from build123d import *

# Parameters (mm, degrees)
SKETCH_W        = 90
SKETCH_H        = 40
PAD_DEPTH       = 11
POCKET_DEPTH    = 9
POCKET001_DEPTH = 6
SKETCH003_W     = 13.5
SKETCH003_H     = 3.4
POCKET002_DEPTH = 6
SKETCH005_R     = 3
HOLE_DEPTH      = 25
FILLET_R        = 1
FILLET001_R     = 2.5
SKETCH007_W     = 6
SKETCH007_H     = 6
POCKET003_DEPTH = 1
FILLET002_R     = 1


with BuildPart() as part:
    # Sketch → Pad (new body)
    with BuildSketch(Plane.XY):
        with Locations((45, 20)):
            Rectangle(SKETCH_W, SKETCH_H)
    extrude(amount=PAD_DEPTH)

    # Sketch001 (on Face6 of Pad) → Pocket (cut)
    with BuildSketch(Plane.XY.offset(11)):
        Polygon((4.5, 30.5), (4.5, 9.5), (9.5, 9.5), (9.5, 4.5), (80.5, 4.5), (80.5, 9.5), (85.5, 9.5), (85.5, 30.5), (80.5, 30.5), (80.5, 35.5), (9.5, 35.5), (9.5, 30.5), align=None)
    extrude(amount=-POCKET_DEPTH, mode=Mode.SUBTRACT)

    # Sketch002 (on Face6 of Pocket) → Pocket001 (cut)
    with BuildSketch(Plane.YZ.offset(90)):
        with BuildLine():
            ThreePointArc((17.5, 11), (20, 8.499988), (22.5, 11))
            Line((17.5, 11), (22.5, 11))
        make_face()
    extrude(amount=-POCKET001_DEPTH, mode=Mode.SUBTRACT)

    # Sketch003 (on Face1 of Pocket001) → Pocket002 (cut)
    with BuildSketch(Plane(origin=(0, 0, 0), x_dir=(0, -1, 0), z_dir=(-1, 0, 0))):
        with Locations((-18.75, 9.3)):
            Rectangle(SKETCH003_W, SKETCH003_H)
    extrude(amount=-POCKET002_DEPTH, mode=Mode.SUBTRACT)

    # Sketch005 (on Face8 of Pocket002) → Hole (cut)
    with BuildSketch(Plane.XY.offset(11)):
        with Locations((4.5, 35.5)):
            Circle(SKETCH005_R)
        with Locations((4.5, 4.5)):
            Circle(SKETCH005_R)
        with Locations((85.5, 35.5)):
            Circle(SKETCH005_R)
        with Locations((85.5, 4.5)):
            Circle(SKETCH005_R)
    extrude(amount=-HOLE_DEPTH, mode=Mode.SUBTRACT)

    # Fillet
    fillet_edges = [part.edges().sort_by_distance(p)[0] for p in [
        (9.5, 30.5, 6.5),
        (80.5, 30.5, 6.5),
        (9.5, 9.5, 6.5),
        (80.5, 9.5, 6.5),
    ]]
    fillet(fillet_edges, radius=FILLET_R)

    # Fillet001
    fillet001_edges = [part.edges().sort_by_distance(p)[0] for p in [
        (0, 40, 5.5),
        (90, 40, 5.5),
        (90, 0, 5.5),
        (0, 0, 5.5),
    ]]
    fillet(fillet001_edges, radius=FILLET001_R)

    # Sketch007 (on Face25 of Fillet001) → Pocket003 (cut)
    with BuildSketch(Plane.XY.offset(2)):
        with Locations((45, 20)):
            Rectangle(SKETCH007_W, SKETCH007_H)
    extrude(amount=-POCKET003_DEPTH, mode=Mode.SUBTRACT)

    # Fillet002
    fillet002_edges = [part.edges().sort_by_distance(p)[0] for p in [
        (48, 23, 1.5),
        (42, 23, 1.5),
        (42, 17, 1.5),
        (48, 17, 1.5),
    ]]
    fillet(fillet002_edges, radius=FILLET002_R)


solid = part.part
The model under review builds one solid part; all positions refer to its coordinate system, in mm. A direction names the side the tool comes from. Round coordinates to 2 decimals unless told otherwise and drop trailing zeros. Write each loop counter-clockwise with the first axis right and the second up, starting at its lowest first coordinate (ties: lowest second). Pieces come first, ordered by that corner, then holes. Notation, with made-up numbers: (87.5, 64) -> (95.5, 64) arc R17 cw to (95.5, 78) -> close; hole circle Ø5 at (78, -16.75). An arc over 180 degrees is marked (long way). Answer as a JSON object with one key per item and string values.
1. We need section D-D on z = 10. State how many separate pieces and enclosed holes the cut face has, and give its area (3 significant figures).
Results found:
{"separate pieces": "2", "enclosed holes": "4", "area": "988 mm^2"}
2. We need section A-A on z = 4.75. State the section outline as (x, y) points, and give its area (3 significant figures).
Results found:
{"outline": "(0, 2.5) arc R2.5 ccw to (2.5, 0) -> (87.5, 0) arc R2.5 ccw to (90, 2.5) -> (90, 37.5) arc R2.5 ccw to (87.5, 40) -> (2.5, 40) arc R2.5 ccw to (0, 37.5) -> close; hole circle Ø6 at (4.5, 4.5); hole circle Ø6 at (4.5, 35.5); hole (4.5, 9.5) -> (8.5, 9.5) arc R1 cw to (9.5, 8.5) -> (9.5, 4.5) -> (80.5, 4.5) -> (80.5, 8.5) arc R1 cw to (81.5, 9.5) -> (85.5, 9.5) -> (85.5, 30.5) -> (81.5, 30.5) arc R1 cw to (80.5, 31.5) -> (80.5, 35.5) -> (9.5, 35.5) -> (9.5, 31.5) arc R1 cw to (8.5, 30.5) -> (4.5, 30.5) -> close; hole circle Ø6 at (85.5, 4.5); hole circle Ø6 at (85.5, 35.5)", "area": "1,070 mm^2"}
3. Machinability: for faces 4 (the face through (2, 25.5, 9)), 5 (the face through (89.248, 39.287, 5.577)), 6 (the face through (83, 9.5, 7)), which of the approach directions +Z, -Z, +X, -X, +Y, -Y give a long, thin tool a straight path to every point of the face, cutting with its end or side? Answer none if there is none.
Results found:
{"face 4": "+Z, -X", "face 5": "+Z, -Z, +X, +Y", "face 6": "+Z"}
4. We need section B-B on y = 20. State the section outline as (x, z) points.
Results found:
{"outline": "(0, 0) -> (90, 0) -> (90, 8.5) -> (85.5, 8.5) -> (85.5, 2) -> (48, 2) -> (48, 1) -> (42, 1) -> (42, 2) -> (4.5, 2) -> (4.5, 7.6) -> (0, 7.6) -> close"}
5. The part is to be moulded in two halves that separate along Y. For faces 1 (the face through (44, 40, 5)), 2 (the face through (45, 4, 11)), 3 (the face through (9.5, 7, 7)), say which applies: pulls with the +Y half, pulls with the -Y half, needs draft (parallel to the pull), parting line crosses it, or undercut.
Results found:
{"face 1": "pulls with the +Y half", "face 2": "needs draft", "face 3": "undercut"}
6. To check wall thickness, follow line 1 along X through (y, z) = (13, 7.5); line 2 along X through (y, z) = (5, 7); line 3 along Y through (x, z) = (75.5, 3.5). State the ranges of each line that lie inside material, in increasing order.
Results found:
{"line 1": "x = 0 to 4.5, 85.5 to 90", "line 2": "x = 0 to 1.54, 7.46 to 9.5, 80.5 to 82.54, 88.46 to 90", "line 3": "y = 0 to 4.5, 35.5 to 40"}
7. We need section C-C on x = 27.5. State the section outline as (y, z) points, and give its area (3 significant figures).
Results found:
{"outline": "(0, 0) -> (40, 0) -> (40, 11) -> (35.5, 11) -> (35.5, 2) -> (4.5, 2) -> (4.5, 11) -> (0, 11) -> close", "area": "161 mm^2"}
8. Clearance check with flat-ended pins moving along their axes: pin 1 (8 mm diameter, centred on x = 4.5, y = 4.5, fed in from +Z); pin 2 (15.5 mm diameter, centred on x = 65, y = 25, fed in from +Z); pin 3 (2 mm diameter, centred on x = 2.5, y = 20, fed in from +Z). State where each tip first meets the part, or that it passes through.
Results found:
{"pin 1": "stops at z = 11", "pin 2": "stops at z = 2", "pin 3": "stops at z = 7.6"}
